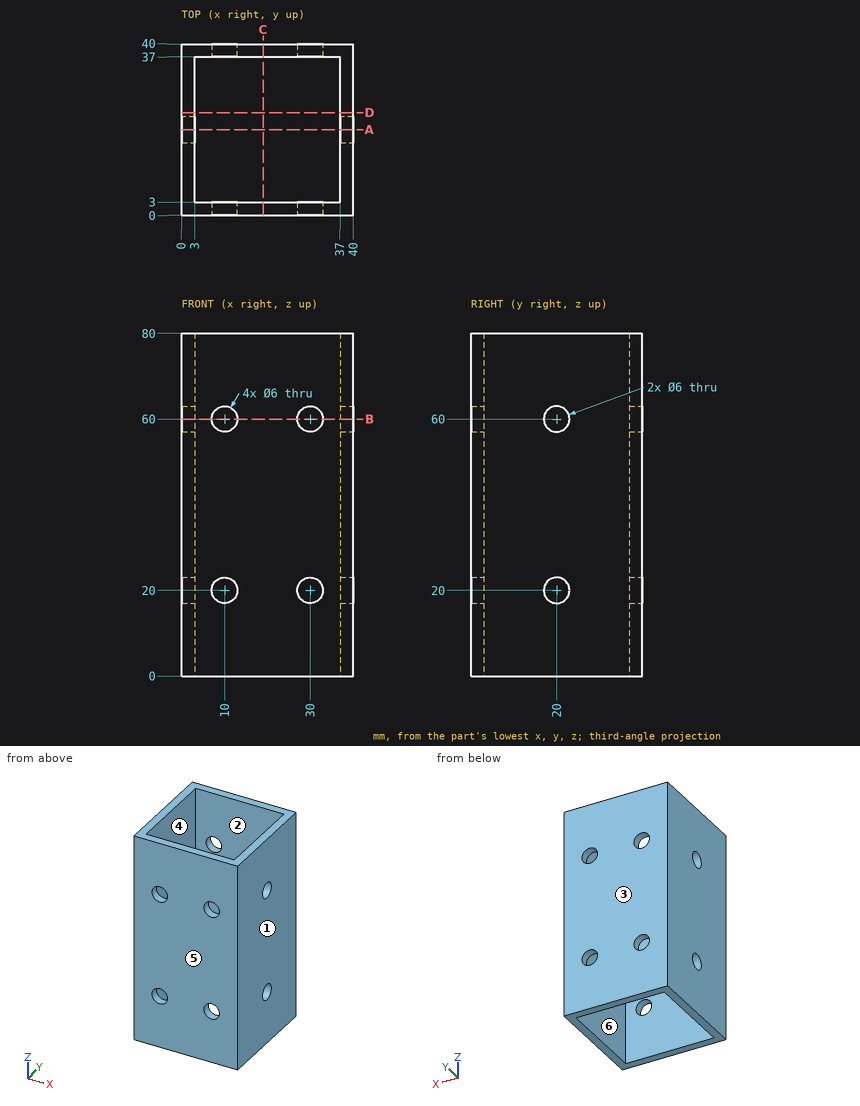
Could you check a few things on this drawing? It's one solid part, dimensions in mm from its lowest x, y, z. A direction names the side the tool comes from. Give positions to 0.01 mm unless a question says otherwise; leave off trailing zeros. Write each loop counter-clockwise with the first axis right and the second up, starting at its lowest first coordinate (ties: lowest second). Pieces come first, ordered by that corner, then holes. Notation, with made-up numbers: (-18, 19) -> (0, 19) arc R30 ccw to (0, 47) -> close; hole circle Ø7 at (-3.5, -22.5). An arc over 180 degrees is marked (long way). Answer as a JSON object with one key per item and string values.
Q1. Suppose I cut it at B-B on z = 60. Count the separate pieces of the cut face and the enclosed holes in it, then the cut area to 3 significant figures.
Taken from the geometry:
{"separate pieces": "6", "enclosed holes": "0", "area": "336 mm²"}
Q2. Suppose I cut it at C-C on x = 19. Write out the boundary of the cut face in (y, z), then the cut area to 3 significant figures.
Taken from the geometry:
{"outline": "(0, 0) -> (3, 0) -> (3, 80) -> (0, 80) -> close; (37, 0) -> (40, 0) -> (40, 80) -> (37, 80) -> close", "area": "480 mm²"}
Q3. Please list where these lines run through material, in increasing order: L1, parallel to Z at x = 2, y = 20; L2, parallel to X at y = 25, z = 72.5.
Taken from the geometry:
{"L1": "z = 0 to 17, 23 to 57, 63 to 80", "L2": "x = 0 to 3, 37 to 40"}
Q4. Which directions (+Z, -Z, +X, -X, +Y, -Y) give clear straight access to the entire face, cutting with the end or side of a thin tool? Please do the marked faces 1 and 2.
Taken from the geometry:
{"face 1": "+Z, -Z, +X, +Y, -Y", "face 2": "+Z, -Z"}
Q5. Suppose I cut it at A-A on y = 20. Write out the boundary of the cut face in (x, z).
Taken from the geometry:
{"outline": "(0, 0) -> (3, 0) -> (3, 17) -> (0, 17) -> close; (0, 23) -> (3, 23) -> (3, 57) -> (0, 57) -> close; (0, 63) -> (3, 63) -> (3, 80) -> (0, 80) -> close; (37, 0) -> (40, 0) -> (40, 17) -> (37, 17) -> close; (37, 23) -> (40, 23) -> (40, 57) -> (37, 57) -> close; (37, 63) -> (40, 63) -> (40, 80) -> (37, 80) -> close"}
Q6. We'd pull the mould along Y, two halves only. Please class the marked faces 3, 4, 5 and 6: released by +Y, released by -Y, zero draft, split by the parting line, or undercut.
Taken from the geometry:
{"face 3": "released by +Y", "face 4": "undercut", "face 5": "released by -Y", "face 6": "undercut"}
